Design review of the part built by this model. Coordinates are the model's own, in mm. A direction names the side the tool comes from. Give positions to 0.01 mm unless a question says otherwise; leave off trailing zeros. Loops run counter-clockwise (first coordinate to the right, second up) from the corner with the lowest first, then second, coordinate; pieces in that order, holes last. Notation, with made-up numbers: (54, 63.25) -> (112, 63.25) arc R3 cw to (112, 68.25) -> close; hole circle Ø8 at (-30, 37.5). An arc over 180 degrees is marked (long way). Answer in a Markdown table with one row per item. Add a question column.
(1) Consider section A-A on x = 0. Write out the cut boundary in (y, z), then the cut area to 3 significant figures.
(2) For pin 1 (10 mm diameter, centred on x = -5, y = -73, fed in from -Z); pin 2 (8 mm diameter, centred on x = -1.5, z = 2, fed in from +Y); pin 3 (4 mm diameter, centred on x = -6, y = -27, fed in from -Z); pin 4 (10 mm diameter, centred on y = -22, z = 2, fed in from -X), all flat-tipped, find the tip position at first contact; note any pin that passes through.
(3) For faces 1 (the flat face through (0, -4, -9.75)), 2 (the flat face through (-4, -6, 4)), list the 3-axis set-ups (+Z, -Z, +X, -X, +Y, -Y) from which the entire face can be reached by the end or side of a thin tool; tool diameter is ignored.
(4) Consider section C-C on y = -50.5. Write out the cut boundary in (x, z), then the cut area to 3 significant figures.
(5) Consider section B-B on z = 0. Write out the cut boundary in (x, y), then the cut area to 3 significant figures.
(6) For line 1 (X direction, y = -64.5, z = -1); line 2 (Z direction, x = -1.25, y = -65.5); line 3 (Y direction, x = -7.75, z = 8.75), list the stretches that pass through material, from the lowest coordinate up.
(7) Consider section D-D on x = 8.75. Write out the cut boundary in (y, z), then the cut area to 3 significant figures.
from build123d import *

# Parameters (mm, degrees)
F0_W     = 19.5
F0_H     = 19.5
F1_DEPTH = 6
F2_R     = 5
F3_DEPTH = 88
F4_SIZE  = 1


with BuildPart() as f1:
    # F0 (on Front) → F1 (new body)
    with BuildSketch(Plane.XZ):
        Rectangle(F0_W, F0_H)
    extrude(amount=F1_DEPTH)

    # F2 (on face) → F3 (join)
    with BuildSketch(Plane.XZ.offset(6)):
        Circle(F2_R)
    extrude(amount=F3_DEPTH)

    # F4
    f4_edges = [f1.edges().sort_by_distance(p)[0] for p in [
        (-5, -94, 0),
    ]]
    chamfer(f4_edges, length=F4_SIZE)

    # F5 (on Top) → F6 (revolve, cut)
    with BuildSketch(Plane.XY):
        with BuildLine():
            ThreePointArc((0, 0), (17.6776695297, -7.3223304703), (25, -25))
            Line((25, -25), (35.5271379938, -25))
            ThreePointArc((35.5271379938, -25), (25.1214801916, 0.1214801916), (0, 10.5271379938))
            Line((0, 10.5271379938), (0, 0))
        make_face()
    revolve(axis=Axis((0, 5.2635689969, 0), (0, -1, 0)), mode=Mode.SUBTRACT)


solid = f1.part
Values follow:
| question | item | result |
|---|---|---|
| 1 | outline | (-94, -4) -> (-93, -5) -> (-6, -5) -> (-6, -9.75) -> (-1.98, -9.75) arc R25 ccw to (-1.98, 9.75) -> (-6, 9.75) -> (-6, 5) -> (-93, 5) -> (-94, 4) -> close |
| 1 | area | 983 mm2 |
| 2 | pin 1 | z = -5 |
| 2 | pin 2 | y = 0 |
| 2 | pin 3 | z = -3 |
| 2 | pin 4 | x = -5 |
| 3 | face 1 | -Z, +X, -X, +Y, -Y |
| 3 | face 2 | -Y |
| 4 | outline | circle Ø10 at (0, 0) |
| 4 | area | 78.5 mm2 |
| 5 | outline | (-9.75, -6) -> (-5, -6) -> (-5, -93) -> (-4, -94) -> (4, -94) -> (5, -93) -> (5, -6) -> (9.75, -6) -> (9.75, -1.98) arc R25 ccw to (-9.75, -1.98) -> close |
| 5 | area | 983 mm2 |
| 6 | line 1 | -4.9 to 4.9 |
| 6 | line 2 | -4.84 to 4.84 |
| 6 | line 3 | -6 to -2.9 |
| 7 | outline | (-6, -9.75) -> (-3.71, -9.75) arc R23.42 ccw to (-3.71, 9.75) -> (-6, 9.75) -> close |
| 7 | area | 72.6 mm2 |
